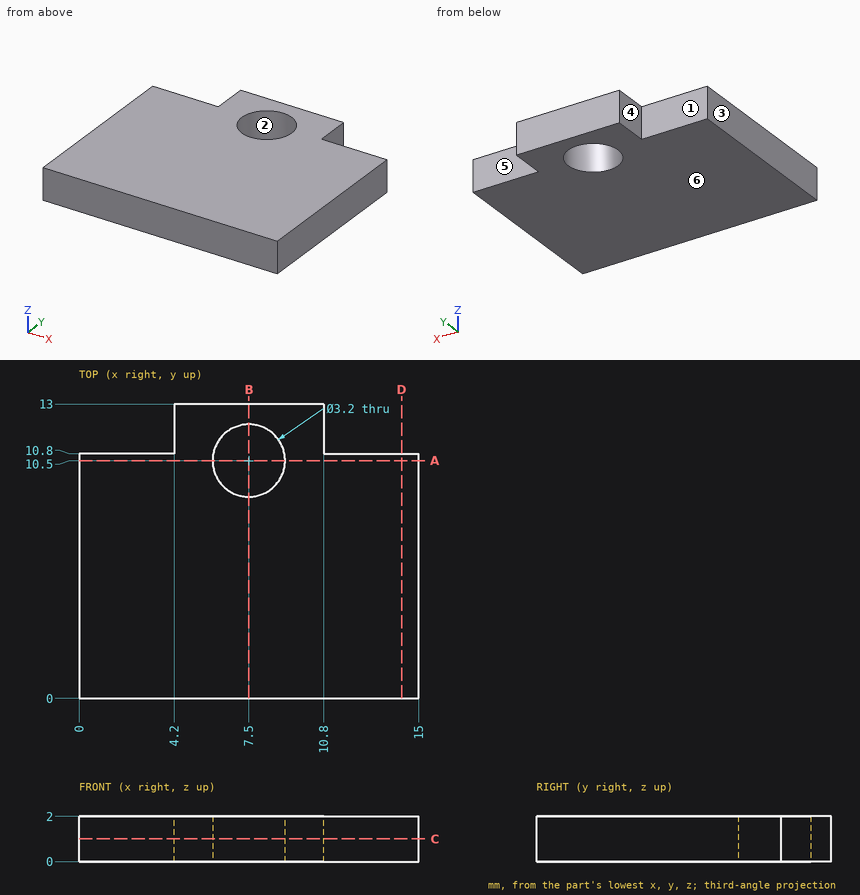
Could you check a few things on this drawing? It's one solid part, dimensions in mm from its lowest x, y, z. A direction names the side the tool comes from. Give positions to 0.01 mm unless a question says otherwise; leave off trailing zeros. Loops run counter-clockwise (first coordinate to the right, second up) from the corner with the lowest first, then second, coordinate; pieces in that order, holes last. Notation, with made-up numbers: (-3.5, 71.5) -> (3.5, 71.5) arc R15 cw to (3.5, 98.5) -> close; hole circle Ø2 at (2.5, -6). An arc over 180 degrees is marked (long way). Answer as CSV lines item,"result". Start each with the question number.
(1) We'd pull the mould along X, two halves only. Please class the marked faces 1, 2 and 3: released by +X, released by -X, zero draft, split by the parting line, or undercut.
(2) If we section it at B-B on x = 7.5: Write out the boundary of the cut face in (y, z), then the cut area to 3 significant figures.
(3) I'm going to push flat-ended pins straight in: pin 1 Ø3 at (x, y) = (7.5, 10.5) entering from -Z; pin 2 Ø1.5 at (x, y) = (8, 7) entering from -Z; pin 3 Ø1 at (y, z) = (11.5, 1) entering from -X; pin 4 Ø1 at (x, z) = (1.5, 1) entering from +Y. Where does each tip first touch, or does it pass through?
(4) If we section it at C-C on z = 1: Write out the boundary of the cut face in (x, y).
(5) If we section it at D-D on x = 14.25: Write out the boundary of the cut face in (y, z), then the cut area to 3 significant figures.
(6) If we section it at A-A on y = 10.5: Write out the boundary of the cut face in (x, z).
(7) Which directions (+Z, -Z, +X, -X, +Y, -Y) give clear straight access to the entire face, cutting with the end or side of a thin tool? Please do the marked faces 4, 5 and 6.
(8) I need wall thicknesses on probe 1 along Y at (x, z) = (7.5, 0.65); probe 2 along Y at (x, z) = (13, 1); probe 3 along Y at (x, z) = (8, 0.6). Which ranges of each line are inside material? Lowest first, please.
Computed:
1,face 1,"zero draft"
1,face 2,"undercut"
1,face 3,"released by -X"
2,outline,"(0, 0) -> (8.9, 0) -> (8.9, 2) -> (0, 2) -> close; (12.1, 0) -> (13, 0) -> (13, 2) -> (12.1, 2) -> close"
2,area,"19.6 mm2"
3,pin 1,"passes through"
3,pin 2,"stops at z = 0"
3,pin 3,"stops at x = 4.2"
3,pin 4,"stops at y = 10.8"
4,outline,"(0, 0) -> (15, 0) -> (15, 10.8) -> (10.8, 10.8) -> (10.8, 13) -> (4.2, 13) -> (4.2, 10.8) -> (0, 10.8) -> close; hole circle Ø3.2 at (7.5, 10.5)"
5,outline,"(0, 0) -> (10.8, 0) -> (10.8, 2) -> (0, 2) -> close"
5,area,"21.6 mm2"
6,outline,"(0, 0) -> (5.9, 0) -> (5.9, 2) -> (0, 2) -> close; (9.1, 0) -> (15, 0) -> (15, 2) -> (9.1, 2) -> close"
7,face 4,"+Z, -Z, -X, +Y"
7,face 5,"+Z, -Z, +X, +Y"
7,face 6,"-Z, +X, -X, +Y, -Y"
8,probe 1,"y = 0 to 8.9, 12.1 to 13"
8,probe 2,"y = 0 to 10.8"
8,probe 3,"y = 0 to 8.98, 12.02 to 13"
